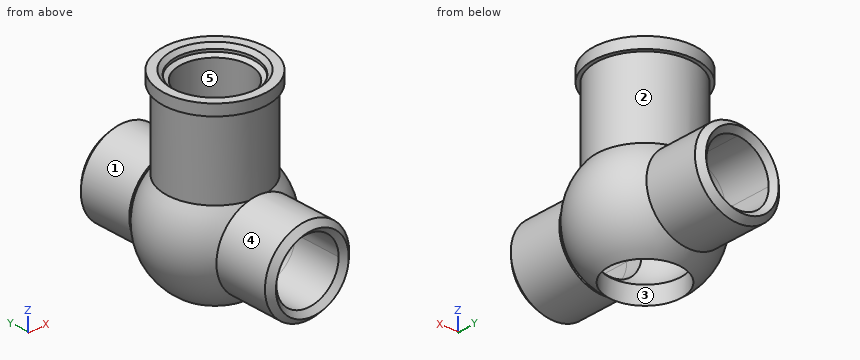
from build123d import *

# Parameters (mm, degrees)
F5_D     = 17
F5_DEPTH = 29
F5_TIP   = 5.1073152617
F6_D     = 17
F6_DEPTH = 29
F6_TIP   = 5.1073152617


with BuildPart() as f2:
    # F0 (on Front) → F2 (revolve)
    with BuildSketch(Plane.XZ):
        with BuildLine():
            Line((-9.3155, 9.5151098654), (-9.3155, 14.2204591962))
            ThreePointArc((-9.3155, 14.2204591962), (-11.2766168332, 12.7215530812), (-13, 10.9544511501))
            ThreePointArc((-13, 10.9544511501), (-16.8567978778, -2.2019003855), (-9.75, -13.9261444772))
            Line((-9.75, -13.9261444772), (-9.75, -9.069363594))
            ThreePointArc((-9.75, -9.069363594), (-13.3123621496, 0.311239453), (-9.3155, 9.5151098654))
        make_face()
        with BuildLine():
            ThreePointArc((-13, 10.9544511501), (-11.2766168332, 12.7215530812), (-9.3155, 14.2204591962))
            Line((-9.3155, 14.2204591962), (-9.3155, 19.2122588888))
            Line((-9.3155, 19.2122588888), (-10.4775, 19.2122588888))
            Line((-10.4775, 19.2122588888), (-10.4775, 33.2122588888))
            Line((-10.4775, 33.2122588888), (-10.55, 33.25))
            Line((-10.55, 33.25), (-10.55, 33.95))
            Line((-10.55, 33.95), (-11.6, 35))
            Line((-11.6, 35), (-14, 35))
            Line((-14, 35), (-14, 32))
            Line((-14, 32), (-13, 32))
            Line((-13, 32), (-13, 10.9544511501))
        make_face()
        Polygon((-10.4775, 19.2122588888), (-9.3155, 19.2122588888), (-9.3155, 32.6073599761), (-10.4775, 33.2122588888), align=None)
    revolve(axis=Axis((0, 0, 10.842), (0, 0, -1)))

    # F1 (on Right) → F3 (revolve)
    with BuildSketch(Plane.YZ):
        with BuildLine():
            Line((27.5668407641, 8.5), (29, 9.9331592359))
            Line((29, 9.9331592359), (27.4331592359, 11.5))
            Line((27.4331592359, 11.5), (12.9851644874, 11.5))
            Line((12.9851644874, 11.5), (12.9851644874, 10.9720327759))
            ThreePointArc((12.9851644874, 10.9720327759), (13.9088267086, 9.7746887209), (14.7224318643, 8.5))
            Line((14.7224318643, 8.5), (27.5668407641, 8.5))
        make_face()
    revolve(axis=Axis((0, 4.3193821889, 0), (0, -1, 0)))

    # F1 (on Right) → F4 (revolve)
    with BuildSketch(Plane.YZ):
        with BuildLine():
            Line((-27.5668407641, 8.5), (-14.7224318643, 8.5))
            ThreePointArc((-14.7224318643, 8.5), (-13.9088267086, 9.7746887209), (-12.9851644874, 10.9720327759))
            Line((-12.9851644874, 10.9720327759), (-12.9851644874, 11.5))
            Line((-12.9851644874, 11.5), (-27.4331592359, 11.5))
            Line((-27.4331592359, 11.5), (-29, 9.9331592359))
            Line((-29, 9.9331592359), (-27.5668407641, 8.5))
        make_face()
    revolve(axis=Axis((0, 4.3193821889, 0), (0, -1, 0)))

    # F5 (one way)
    with BuildSketch(Plane(origin=(0, 0, 0), x_dir=(1, 0, 0), z_dir=(0, 1, 0))):
        with Locations((0, 0)):
            Circle(F5_D / 2)
    extrude(amount=-F5_DEPTH, mode=Mode.SUBTRACT)
    with Locations(Plane(origin=(0, 0, 0), x_dir=(1, 0, 0), z_dir=(0, 1, 0))):
        with Locations((0, 0)):
            with Locations((0, 0, -(F5_DEPTH + F5_TIP / 2))):  # 118° drill point
                Cone(0, F5_D / 2, F5_TIP, mode=Mode.SUBTRACT)

    # F6
    with Locations(Plane.XZ):
        with Locations((0, 0)):
            Hole(F6_D / 2, depth=F6_DEPTH)
            with Locations((0, 0, -(F6_DEPTH + F6_TIP / 2))):  # 118° drill point
                Cone(0, F6_D / 2, F6_TIP, mode=Mode.SUBTRACT)


solid = f2.part
Could you check a few things on this model? Use its own coordinates, in mm. Face numbers are marked on the shaded views. A direction names the side the tool comes from. Coordinates: 2 decimals unless noted, no trailing zeros. Order: outer loops, then holes, each group sorted by start corner. A loop starts at its lowest first (then second) coordinate and runs counter-clockwise, first axis right, second up.
Q1. Suppose I cut it at B-B on x = 6. Give the number of separate pieces and of enclosed holes in the cut face, and give its area (3 significant figures).
Q2. Suppose I cut it at C-C on y = 24. Please give me the cut outline in (x, z).
Q3. Please list where these lines run through material, in increasing order: L1, parallel to Z at x = 0, y = 23; L2, parallel to Y at x = -3.5, z = 25.
Q4. Will these pins go through, and if not, where does the flat tip stop? pin 1 (3 mm diameter, centred on x = 0, y = 17.5, fed in from +Z); pin 2 (11.5 mm diameter, centred on x = 1, z = 4, fed in from -Y); pin 3 (5 mm diameter, centred on x = 5.5, z = 12, fed in from +Y); pin 4 (8.5 mm diameter, centred on x = 6, y = 2.5, fed in from -Z).
Q5. Which directions (+Z, -Z, +X, -X, +Y, -Y) give clear straight access to the entire face, cutting with the end or side of a thin tool? Please do the marked faces 1, 2 and 3.
Q6. Thinking about a two-plate mould opening in Y: for the marked faces 4 and 5, which applies, released by +Y, released by -Y, zero draft, split by the parting line, or undercut?
Q7. Suppose I cut it at A-A on z = 13.5. Please give me the cut outline in (x, y), and give its area (3 significant figures).
Answer:
1. separate pieces: 4
1. enclosed holes: 0
1. area: 539 mm2
2. outline: circle Ø23 at (0, 0); hole circle Ø17 at (0, 0)
3. L1: z = -11.5 to -8.5, 8.5 to 11.5
3. L2: y = -12.52 to -8.63, 8.63 to 12.52
4. pin 1: stops at z = 11.5
4. pin 2: stops at y = -28.94
4. pin 3: stops at y = 28.23
4. pin 4: stops at z = -13.93
5. face 1: +Y
5. face 2: none
5. face 3: -Z
6. face 4: zero draft
6. face 5: undercut
7. outline: circle Ø26 at (0, 0); hole circle Ø18.63 at (0, 0)
7. area: 258 mm2
